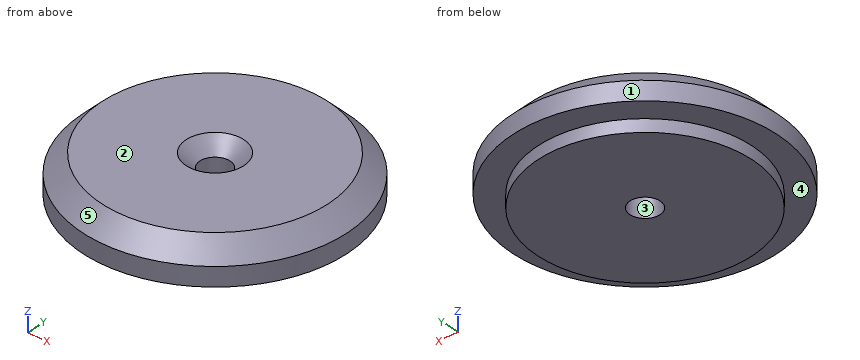
Solid Edge part; units mm, degrees
sketch "Sketch1" plane through (0, 0, 0) normal (0, -1, 0) x (1, 0, 0)
  line L0 (0, 0) -> (17, 0)
  line L1 (17, 0) -> (17, 2)
  line L2 (17, 2) -> (21, 2)
  line L3 (21, 2) -> (21, 8)
  line L4 (21, 8) -> (0, 8)
  dimension "D1" = 21
revolve "RevolvedProtrusion1" add sketch "Sketch1" angle 360 about axis through (0, 0, 10) along (0, 0, -1)
chamfer "Chamfer1" distance 3 angle 45 1 edges at (-21, 0, 8)
hole "Hole_1" at (0, 0, 8) direction (0, 0, -1) diameter 4.8 end up to next countersink diameter 9.18 countersink angle 90
properties material "Polyethylene, low density"
Could you check a few things on this model? Use its own coordinates, in mm. Face numbers are marked on the shaded views. A direction names the side the tool comes from. Give positions to 0.01 mm unless a question says otherwise; leave off trailing zeros. Write each loop counter-clockwise with the first axis right and the second up, starting at its lowest first coordinate (ties: lowest second). Pieces come first, ordered by that corner, then holes. Notation, with made-up numbers: (61, 21) - (117, 21) arc R21 ccw to (117, 46) - close; hole circle Ø10 at (29, 2). An arc over 180 degrees is marked (long way). One line per item, written item: value. Start each with the question number.
Item 1: Imagine slicing it at A-A, the plane y = 0. List the corners of the cut face in (x, z) for me, and give its area (3 significant figures).
Item 2: Please list where these lines run through material, in increasing order: line 1 (X direction, y = 0, z = 1.85); line 2 (X direction, y = 0, z = 4.15). Write a range as from..to.
Item 3: If we mould it in two halves opening along Y, with no side actions, what happens to the marked faces 1, 2 and 3? For each: +Y half, -Y half, draft (parallel to the pull), parting line (faces both ways), or undercut.
Item 4: I'm going to push flat-ended pins straight in: pin 1 (2 mm diameter, centred on y = 15.5, z = 7, fed in from -X); pin 2 (1.5 mm diameter, centred on y = -3.5, z = 2, fed in from +X); pin 3 (5 mm diameter, centred on x = 11.5, y = 13, fed in from -Z); pin 4 (4 mm diameter, centred on x = 4, z = 3.5, fed in from -Y). Where does each tip first touch, or does it pass through?
Item 5: Imagine slicing it at D-D, the plane z = 2.5. List the corners of the cut face in (x, y) for me, and give its area (3 significant figures).
Item 6: Imagine slicing it at C-C, the plane z = 7.25. List the corners of the cut face in (x, y) for me, and give its area (3 significant figures).
Item 7: Which directions (+Z, -Z, +X, -X, +Y, -Y) give clear straight access to the entire face, cutting with the end or side of a thin tool? Please do the marked faces 4 and 5.
Geometry says:
1. outline: (-21, 2) - (-17, 2) - (-17, 0) - (-2.4, 0) - (-2.4, 5.81) - (-4.59, 8) - (-18, 8) - (-21, 5) - close; (2.4, 0) - (17, 0) - (17, 2) - (21, 2) - (21, 5) - (18, 8) - (4.59, 8) - (2.4, 5.81) - close
1. area: 268 mm^2
2. line 1: -17..-2.4, 2.4..17
2. line 2: -21..-2.4, 2.4..21
3. face 1: parting line
3. face 2: draft
3. face 3: undercut
4. pin 1: x = -13.04
4. pin 2: x = 20.82
4. pin 3: z = 0
4. pin 4: y = -20.9
5. outline: circle Ø42 at (0, 0); hole circle Ø4.8 at (0, 0)
5. area: 1,370 mm^2
6. outline: circle Ø37.5 at (0, 0); hole circle Ø7.68 at (0, 0)
6. area: 1,060 mm^2
7. face 4: -Z
7. face 5: +Z
